Could you check a few things on this model? Use its own coordinates, in mm. Round coordinates to 2 decimals unless told otherwise and drop trailing zeros. Loops run counter-clockwise (first coordinate to the right, second up) from the corner with the lowest first, then second, coordinate; pieces in that order, holes last. Notation, with made-up numbers: M 3,88 L 20,88 A20 ccw 20,94 Z; hole C -17.5,86 d7. An arc over 180 degrees is marked long. Answer in a Markdown table with one row per item.
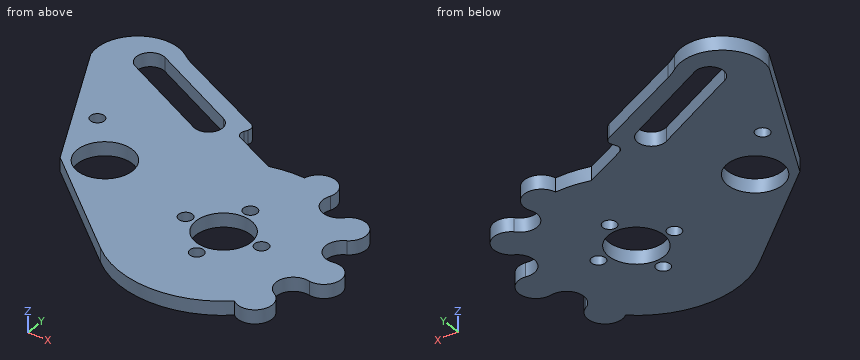
```python
from build123d import *

# Parameters (mm, degrees)
ESQUISSE1_R        = 4
ESQUISSE1_R_2      = 1
BOSS_EXTRU_1_DEPTH = 2
CONG_1_R           = 1
CONG_2_R           = 11


with BuildPart() as part:
    # Esquisse1 → Boss.-Extru.1 (new body)
    with BuildSketch(Plane.XY):
        with BuildLine():
            Line((-3.728432128, 14.529239273), (-10.902133324, 18.092613259))
            Line((-10.902133324, 18.092613259), (-9.77414371, 20.363455577))
            Line((-9.77414371, 20.363455577), (-25.005281494, 27.929179137))
            ThreePointArc((-25.005281494, 27.929179137), (-32.144223962, 28.809157948), (-34.856074883, 22.146971607))
            Line((-34.856074883, 22.146971607), (-25.005281494, 1.884444499))
            Line((-25.005281494, 1.884444499), (-9.850606554, -11.31218593))
            ThreePointArc((-9.850606554, -11.31218593), (-0.12474397, -14.999481289), (9.661100255, -11.47445606))
            ThreePointArc((9.661100255, -11.47445606), (13.285456142, -11.120563185), (12.711512496, -7.524484146))
            ThreePointArc((12.711512496, -7.524484146), (11.513856086, -4.40486723), (14.487891216, -2.881218443))
            ThreePointArc((14.487891216, -2.881218443), (17.321259352, -0.471730027), (14.623234656, 2.088401251))
            ThreePointArc((14.623234656, 2.088401251), (11.736537034, 3.771662198), (13.102212542, 6.821468911))
            ThreePointArc((13.102212542, 6.821468911), (13.803708164, 10.474072546), (10.097110191, 10.781872629))
            ThreePointArc((10.097110191, 10.781872629), (6.792233583, 10.287725708), (5.948313856, 13.521019705))
            ThreePointArc((5.948313856, 13.521019705), (4.31988032, 16.778227095), (1.167882396, 14.954465912))
            ThreePointArc((1.167882396, 14.954465912), (-1.297808983, 14.94375093), (-3.728432128, 14.529239273))
        make_face()
        with Locations((-20.325227829, 4.439090716)):
            Circle(ESQUISSE1_R, mode=Mode.SUBTRACT)
        with Locations((-26.256387143, 11.319323515)):
            Circle(ESQUISSE1_R_2, mode=Mode.SUBTRACT)
        with BuildLine():
            ThreePointArc((-29.058075564, 23.063121212), (-29.928943128, 25.754141406), (-27.237922934, 26.625008971))
            Line((-27.237922934, 26.625008971), (-14.025891569, 19.873557138))
            ThreePointArc((-14.025891569, 19.873557138), (-13.155024005, 17.182536944), (-15.846044199, 16.31166938))
            Line((-15.846044199, 16.31166938), (-29.058075564, 23.063121212))
        make_face(mode=Mode.SUBTRACT)
        with Locations((5.5, 0)):
            Circle(ESQUISSE1_R_2, mode=Mode.SUBTRACT)
        with Locations((0, -5.5)):
            Circle(ESQUISSE1_R_2, mode=Mode.SUBTRACT)
        with Locations((-5.5, 0)):
            Circle(ESQUISSE1_R_2, mode=Mode.SUBTRACT)
        Circle(ESQUISSE1_R, mode=Mode.SUBTRACT)
        with Locations((0, 5.5)):
            Circle(ESQUISSE1_R_2, mode=Mode.SUBTRACT)
    extrude(amount=BOSS_EXTRU_1_DEPTH)

    # Congé1
    cong_1_edges = [part.edges().sort_by_distance(p)[0] for p in [
        (-9.77414371, 20.363455577, 1),
        (-10.902133324, 18.092613259, 1),
    ]]
    fillet(cong_1_edges, radius=CONG_1_R)

    # Congé2
    cong_2_edges = [part.edges().sort_by_distance(p)[0] for p in [
        (-25.005281494, 27.929179137, 1),
    ]]
    fillet(cong_2_edges, radius=CONG_2_R)


solid = part.part
```
1) I want a section at C-C, the plane z = 0.6. State how many separate pieces and enclosed holes the cut face has, plus the area to 3 significant figures.
Computed:
| item | result |
|---|---|
| separate pieces | 1 |
| enclosed holes | 8 |
| area | 1,060 mm² |
2) I want a section at D-D, the plane x = -5.5. Please give me the cut outline in (y, z), plus the area to 3 significant figures.
Computed:
| item | result |
|---|---|
| outline | M -13.96,0 L -1,0 L -1,2 L -13.96,2 Z; M 1,0 L 15.41,0 L 15.41,2 L 1,2 Z |
| area | 54.7 mm² |
3) Will these pins go through, and if not, where does the flat tip stop? P1, Ø1.2, axis at x = 5.5, y = 0, coming from the +Z side; P2, Ø2.5, axis at x = 0, y = -5.5, coming from the +Z side; P3, Ø1, axis at x = 4, z = 1, coming from the +Y side.
Computed:
| item | result |
|---|---|
| P1 | passes through |
| P2 | stops at z = 2 |
| P3 | stops at y = 16.88 |
4) I want a section at A-A, the plane x = 0. Please give me the cut outline in (y, z), plus the area to 3 significant figures.
Computed:
| item | result |
|---|---|
| outline | M -15,0 L -6.5,0 L -6.5,2 L -15,2 Z; M -4.5,0 L -4,0 L -4,2 L -4.5,2 Z; M 4,0 L 4.5,0 L 4.5,2 L 4,2 Z; M 6.5,0 L 15,0 L 15,2 L 6.5,2 Z |
| area | 36.0 mm² |
5) I want a section at B-B, the plane y = -5.5. Please give me the cut outline in (x, z).
Computed:
| item | result |
|---|---|
| outline | M -16.53,0 L -1,0 L -1,2 L -16.53,2 Z; M 1,0 L 11.36,0 L 11.36,2 L 1,2 Z |
6) I need wall thicknesses on line 1 (Y direction, x = 0, z = 1.25); line 2 (Y direction, x = -23.5, z = 1.5); line 3 (Y direction, x = -17, z = 1.3). Which ranges of each line are inside material? Lowest first, please.
Computed:
| item | result |
|---|---|
| line 1 | y = -15 to -6.5, -4.5 to -4, 4 to 4.5, 6.5 to 15 |
| line 2 | y = 0.57 to 2.01, 6.87 to 20.22, 24.71 to 27.18 |
| line 3 | y = -5.09 to 2.22, 6.66 to 16.9, 21.39 to 23.95 |
